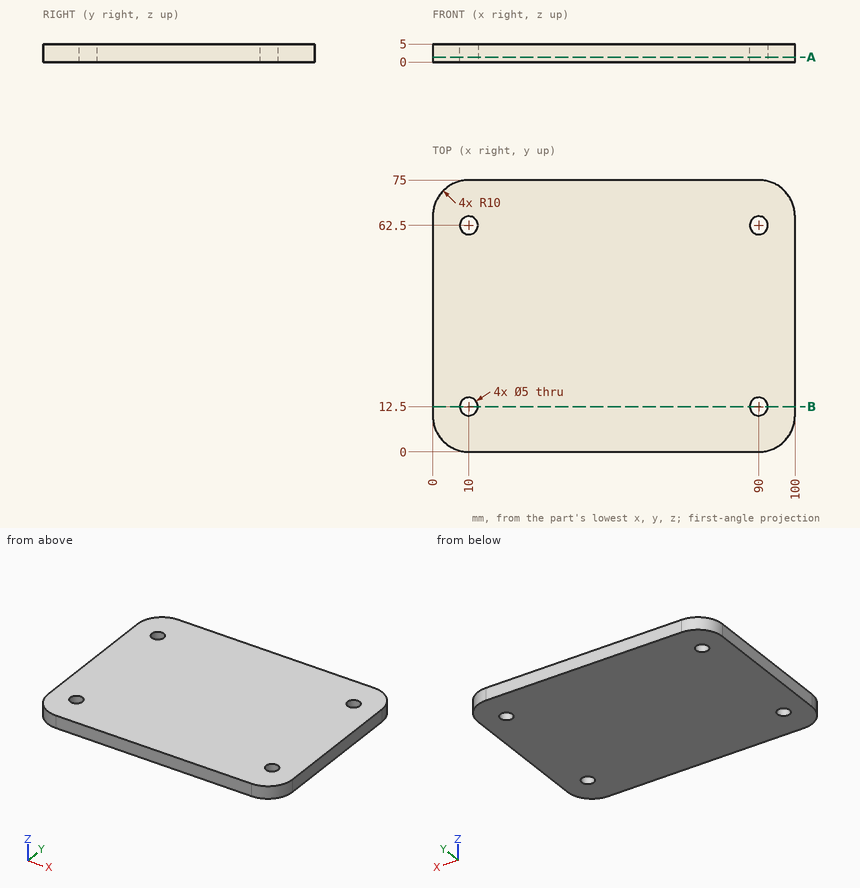
Can you work these out from the drawing? Everything is in mm from the part's minimum corner. Give positions to 0.01 mm unless a question says otherwise; leave off trailing zeros. Order: outer loops, then holes, each group sorted by start corner. A loop starts at its lowest first (then second) coordinate and runs counter-clockwise, first axis right, second up. Notation, with made-up numbers: M -27,74 L -14,74 A19 ccw -14,102 Z; hole C 83.5,16 d8. An arc over 180 degrees is marked long. One line per question, with ' | ' between items.
1. If I drill on line 1 (Y direction, x = 90, z = 3.85); line 2 (X direction, y = 12, z = 2.3); line 3 (Y direction, x = 94.5, z = 1.3), over which ranges is the centre line in solid material (lowest first)?
Results:
line 1: 0 to 10, 15 to 60, 65 to 75 | line 2: 0 to 7.55, 12.45 to 87.55, 92.45 to 100 | line 3: 1.07 to 73.93
2. I want a section at A-A (z = 1.4). List the corners of the cut face in (x, y) for me.
Results:
outline: M 0,10 A10 ccw 10,0 L 90,0 A10 ccw 100,10 L 100,65 A10 ccw 90,75 L 10,75 A10 ccw 0,65 Z; hole C 10,12.5 d5; hole C 10,62.5 d5; hole C 90,12.5 d5; hole C 90,62.5 d5
3. I'm going to push a flat-ended pin straight in: pin 1 (6.5 mm diameter, centred on x = 90, y = 62.5, fed in from -Z). Where does the tip first touch, or does it pass through?
Results:
pin 1: z = 0
4. I want a section at B-B (y = 12.5). List the corners of the cut face in (x, z) for me.
Results:
outline: M 0,0 L 7.5,0 L 7.5,5 L 0,5 Z; M 12.5,0 L 87.5,0 L 87.5,5 L 12.5,5 Z; M 92.5,0 L 100,0 L 100,5 L 92.5,5 Z
